Source: CAD feature listing. Evaluate the final solid. Frame: model axes, mm. A direction names the side the tool comes from. Round coordinates to 2 decimals unless told otherwise and drop trailing zeros. Loops run counter-clockwise (first coordinate to the right, second up) from the corner with the lowest first, then second, coordinate; pieces in that order, holes last. Notation, with made-up numbers: (20, 38.25) - (78, 38.25) arc R17 cw to (78, 60.25) - close; hole circle Ø1 at (78, -34.75). An arc over 180 degrees is marked (long way). One line per question, with ' | ' between items. Start each with the question number.
1. Mould query, pull axis Z, two halves, no side actions, for faces 5 (the flat face through (4.93, 20.985, -17.465)), 6 (the flat face through (12.218, -3.979, -5.393)), 7 (the flat face through (12, -7.7, 0)). Classes: pulls with the +Z half, pulls with the -Z half, needs draft (parallel to the pull), parting line crosses it, or undercut.
2. Ray query, line 1 (Z direction, x = 1.15, y = 0); line 2 (Y direction, x = 9, z = 13); line 3 (Z direction, x = 10.25, y = 1.5). Return the intervals inside material, ascending.
3. Cut plane D-D (x = 1). Return loops of the section in (y, z).
4. Cut plane B-B (y = 0). Return loops of the section in (x, z), then the cut area to 4 significant figures.
5. Cut plane C-C (y = -16.5). Return loops of the section in (x, z).
6. Cut plane A-A (z = 0). Return loops of the section in (x, y).
7. Pin query (flat end, axial travel): pin 1 (1.3 mm diameter, centred on x = 13, z = -1.5, fed in from +Y); pin 2 (1.4 mm diameter, centred on x = 12.5, z = -7.5, fed in from +Y); pin 3 (6 mm diameter, centred on x = 13.5, y = 9, fed in from -Z). Return the tip coordinate at first contact, or that it passes through.
8. Access query for faces 1 (the flat face through (8, -16, 17.5)), 2 (the flat face through (12, 7, 5)), 3 (the flat face through (2, -16, 15)), 4 (the flat face through (12, -5, -7)). Directions: +Z, -Z, +X, -X, +Y, -Y. A direction counts if a zero-diameter tool reaches every point of the face in a straight line with its end or side. Return the directions, or none.
```python
from build123d import *

# Parameters (mm, degrees)
F0_W      = 46.9
F0_H      = 40
F1_DEPTH  = 10
F2_SIZE   = 5
F4_DEPTH  = 5
F5_SIZE   = 0.5
F6_R      = 5
F6_R_2    = 2.5
F7_DEPTH  = 5
F8_DEPTH  = 15.001
F10_DEPTH = 5


with BuildPart() as f1:
    # F0 (on Right) → F1 (new body)
    with BuildSketch(Plane.YZ):
        Rectangle(F0_W, F0_H)
        with BuildLine():
            Line((-14.7, -15), (-17.2, -15))
            ThreePointArc((-17.2, -15), (-19.7, -12.5), (-17.2, -10))
            Line((-17.2, -10), (-14.7, -10))
            ThreePointArc((-14.7, -10), (-12.2, -12.5), (-14.7, -15))
        make_face(mode=Mode.SUBTRACT)
        with BuildLine():
            ThreePointArc((14.7, -15), (12.2, -12.5), (14.7, -10))
            Line((14.7, -10), (17.2, -10))
            ThreePointArc((17.2, -10), (19.7, -12.5), (17.2, -15))
            Line((17.2, -15), (14.7, -15))
        make_face(mode=Mode.SUBTRACT)
        with BuildLine():
            ThreePointArc((-14.7, 15), (-12.2, 12.5), (-14.7, 10))
            Line((-14.7, 10), (-17.2, 10))
            ThreePointArc((-17.2, 10), (-19.7, 12.5), (-17.2, 15))
            Line((-17.2, 15), (-14.7, 15))
        make_face(mode=Mode.SUBTRACT)
        with BuildLine():
            Line((17.2, 10), (14.7, 10))
            ThreePointArc((14.7, 10), (12.2, 12.5), (14.7, 15))
            Line((14.7, 15), (17.2, 15))
            ThreePointArc((17.2, 15), (19.7, 12.5), (17.2, 10))
        make_face(mode=Mode.SUBTRACT)
    extrude(amount=F1_DEPTH)

    # F2
    f2_edges = [f1.edges().sort_by_distance(p)[0] for p in [
        (5, -23.45, -20),
        (5, -23.45, 20),
        (5, 23.45, -20),
        (5, 23.45, 20),
    ]]
    chamfer(f2_edges, length=F2_SIZE)

    # F3 (on face) → F4 (join)
    with BuildSketch(Plane.YZ.offset(10)):
        Polygon((0, 4.4), (2.9857864376, 4.4), (5, 6.4142135624), (5, 7.7), (-5, 7.7), (-5, 6.4142135624), (-2.9857864376, 4.4), align=None)
        Polygon((-7.7, 5), (-7.7, -5), (-6.4142135624, -5), (-4.4, -2.9857864376), (-4.4, 0), (-4.4, 2.9857864376), (-6.4142135624, 5), align=None)
        Polygon((-5, -7.7), (5, -7.7), (5, -6.4142135624), (2.9857864376, -4.4), (0, -4.4), (-2.9857864376, -4.4), (-5, -6.4142135624), align=None)
        Polygon((7.7, -5), (7.7, 5), (6.4142135624, 5), (4.4, 2.9857864376), (4.4, 0), (4.4, -2.9857864376), (6.4142135624, -5), align=None)
    extrude(amount=F4_DEPTH)

    # F5
    f5_edges = [f1.edges().sort_by_distance(p)[0] for p in [
        (15, -5, -7.057107),
        (15, 0, -7.7),
        (15, 5, -7.057107),
        (15, 3.992893, -5.407107),
        (15, 0, -4.4),
        (15, -3.992893, -5.407107),
        (15, -7.057107, 5),
        (15, -7.7, 0),
        (15, -7.057107, -5),
        (15, -5.407107, -3.992893),
        (15, -4.4, 0),
        (15, -5.407107, 3.992893),
        (15, 0, 4.4),
        (15, 3.992893, 5.407107),
        (15, 5, 7.057107),
        (15, 0, 7.7),
        (15, -5, 7.057107),
        (15, -3.992893, 5.407107),
        (15, 4.4, 0),
        (15, 5.407107, -3.992893),
        (15, 7.057107, -5),
        (15, 7.7, 0),
        (15, 7.057107, 5),
        (15, 5.407107, 3.992893),
    ]]
    chamfer(f5_edges, length=F5_SIZE)

    # F6 (on face) → F7 (cut)
    with BuildSketch(Plane(origin=(0, 0, 0), x_dir=(0, -1, 0), z_dir=(-1, 0, 0))):
        Circle(F6_R)
        Circle(F6_R_2, mode=Mode.SUBTRACT)
    extrude(amount=-F7_DEPTH, mode=Mode.SUBTRACT)

    # F8 (cut, through all): a face of the model
    f8_faces = [f1.faces().sort_by_distance(p)[0] for p in [
        (0, 0, 0),
    ]]
    extrude(f8_faces, amount=-F8_DEPTH, mode=Mode.SUBTRACT)

    # F9 (on face) → F10 (cut)
    with BuildSketch(Plane.YZ.offset(10)):
        with BuildLine():
            ThreePointArc((17.2, 7.5), (22.2, 12.5), (17.2, 17.5))
            Line((17.2, 17.5), (14.7, 17.5))
            ThreePointArc((14.7, 17.5), (9.7, 12.5), (14.7, 7.5))
            Line((14.7, 7.5), (17.2, 7.5))
        make_face()
        with BuildLine():
            ThreePointArc((-14.7, 7.5), (-9.7, 12.5), (-14.7, 17.5))
            Line((-14.7, 17.5), (-17.2, 17.5))
            ThreePointArc((-17.2, 17.5), (-22.2, 12.5), (-17.2, 7.5))
            Line((-17.2, 7.5), (-14.7, 7.5))
        make_face()
        with BuildLine():
            ThreePointArc((-17.2, -7.5), (-22.2, -12.5), (-17.2, -17.5))
            Line((-17.2, -17.5), (-14.7, -17.5))
            ThreePointArc((-14.7, -17.5), (-9.7, -12.5), (-14.7, -7.5))
            Line((-14.7, -7.5), (-17.2, -7.5))
        make_face()
        with BuildLine():
            ThreePointArc((14.7, -7.5), (9.7, -12.5), (14.7, -17.5))
            Line((14.7, -17.5), (17.2, -17.5))
            ThreePointArc((17.2, -17.5), (22.2, -12.5), (17.2, -7.5))
            Line((17.2, -7.5), (14.7, -7.5))
        make_face()
    extrude(amount=-F10_DEPTH, mode=Mode.SUBTRACT)


solid = f1.part
```
Answers follow:
1) face 5: pulls with the -Z half | face 6: undercut | face 7: needs draft
2) line 1: z = -20 to -5, 5 to 20 | line 2: y = -23.45 to -22.17, -9.73 to 9.73, 22.17 to 23.45 | line 3: z = -7.7 to -4.4, 4.4 to 7.7
3) outline: (-23.45, -15) - (-18.45, -20) - (18.45, -20) - (23.45, -15) - (23.45, 15) - (18.45, 20) - (-18.45, 20) - (-23.45, 15) - close; hole (-17.2, -15) - (-14.7, -15) arc R2.5 ccw to (-14.7, -10) - (-17.2, -10) arc R2.5 ccw to start; hole (-17.2, 10) - (-14.7, 10) arc R2.5 ccw to (-14.7, 15) - (-17.2, 15) arc R2.5 ccw to start; hole circle Ø10 at (0, 0); hole (14.7, -15) - (17.2, -15) arc R2.5 ccw to (17.2, -10) - (14.7, -10) arc R2.5 ccw to start; hole (14.7, 10) - (17.2, 10) arc R2.5 ccw to (17.2, 15) - (14.7, 15) arc R2.5 ccw to start
4) outline: (0, -20) - (10, -20) - (10, -7.7) - (14.5, -7.7) - (15, -7.2) - (15, -4.9) - (14.5, -4.4) - (10, -4.4) - (10, -2.5) - (5, -2.5) - (5, -5) - (0, -5) - close; (0, 5) - (5, 5) - (5, 2.5) - (10, 2.5) - (10, 4.4) - (14.5, 4.4) - (15, 4.9) - (15, 7.2) - (14.5, 7.7) - (10, 7.7) - (10, 20) - (0, 20) - close | area: 357.5 mm2
5) outline: (0, -20) - (10, -20) - (10, -17.5) - (5, -17.5) - (5, -15) - (0, -15) - close; (0, -10) - (5, -10) - (5, -7.5) - (10, -7.5) - (10, 7.5) - (5, 7.5) - (5, 10) - (0, 10) - close; (0, 15) - (5, 15) - (5, 17.5) - (10, 17.5) - (10, 20) - (0, 20) - close
6) outline: (0, -23.45) - (10, -23.45) - (10, -7.7) - (14.5, -7.7) - (15, -7.2) - (15, -4.9) - (14.5, -4.4) - (10, -4.4) - (10, -2.5) - (5, -2.5) - (5, -5) - (0, -5) - close; (0, 5) - (5, 5) - (5, 2.5) - (10, 2.5) - (10, 4.4) - (14.5, 4.4) - (15, 4.9) - (15, 7.2) - (14.5, 7.7) - (10, 7.7) - (10, 23.45) - (0, 23.45) - close
7) pin 1: stops at y = 7.7 | pin 2: stops at y = 5 | pin 3: stops at z = -5
8) face 1: +X | face 2: +Z, +X, +Y | face 3: +X, -X | face 4: -Z, +X, -Y
